Could you check a few things on this drawing? It's one solid part, dimensions in mm from its lowest x, y, z. A direction names the side the tool comes from. Coordinates: 2 decimals unless noted, no trailing zeros. Loops run counter-clockwise (first coordinate to the right, second up) from the corner with the lowest first, then second, coordinate; pieces in that order, holes last.
1) For the marked faces 1, 2 and 3, which set-ups out of +Z, -Z, +X, -X, +Y, -Y let a thin tool reach every point of the face, with its end or its side?
2) Will these pins go through, and if not, where does the flat tip stop? P1, Ø2, axis at y = 12.5, z = 1, coming from the +X side (1 decimal); P2, Ø1, axis at y = 7.5, z = 1.5, coming from the -X side (1 decimal).
3) Imagine slicing it at D-D on x = 0.5. Please give me the cut outline in (y, z) (1 decimal).
4) Imagine slicing it at A-A on x = 5.25. Please give me the cut outline in (y, z).
5) Imagine slicing it at B-B on z = 2.5. Please give me the cut outline in (x, y).
6) If I drill on line 1 along Y through (x, z) = (5, 0.5); line 2 along Z through (x, y) = (2.25, 10); line 3 along X through (y, z) = (18.25, 6) (1 decimal), over which ranges is the centre line in solid material (lowest first)?
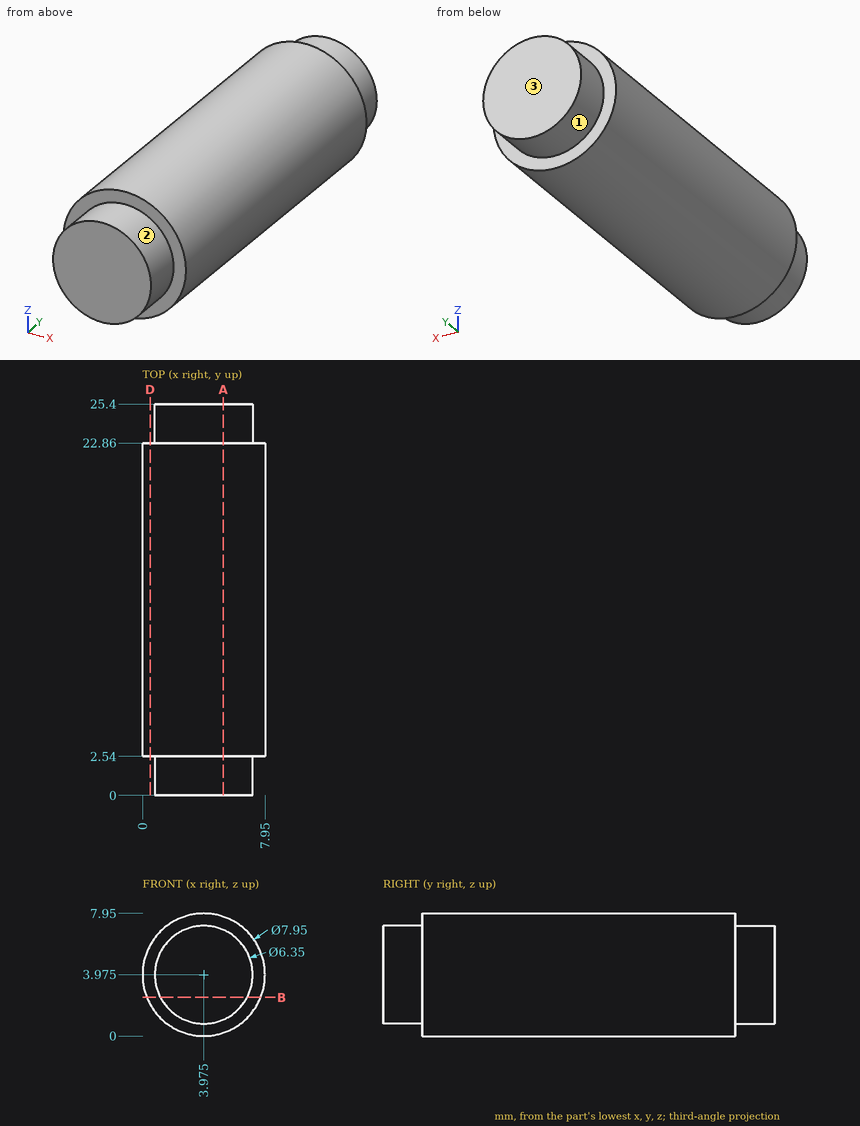
Filled in:
1. face 1: +Y
1. face 2: -Y
1. face 3: +Z, -Z, +X, -X, +Y
2. P1: stops at x = 7.4
2. P2: stops at x = 0.5
3. outline: (2.5, 2) - (22.9, 2) - (22.9, 5.9) - (2.5, 5.9) - close
4. outline: (0, 1.07) - (2.54, 1.07) - (2.54, 0.21) - (22.86, 0.21) - (22.86, 1.07) - (25.4, 1.07) - (25.4, 6.88) - (22.86, 6.88) - (22.86, 7.74) - (2.54, 7.74) - (2.54, 6.88) - (0, 6.88) - close
5. outline: (0.28, 2.54) - (1.16, 2.54) - (1.16, 0) - (6.79, 0) - (6.79, 2.54) - (7.67, 2.54) - (7.67, 22.86) - (6.79, 22.86) - (6.79, 25.4) - (1.16, 25.4) - (1.16, 22.86) - (0.28, 22.86) - close
6. line 1: y = 2.54 to 22.86
6. line 2: z = 0.39 to 7.56
6. line 3: x = 0.6 to 7.4
